Here's how the part is built. I have some questions about the finished solid (model axes, mm). Coordinates: 2 decimals unless noted, no trailing zeros. Write each loop counter-clockwise with the first axis right and the second up, starting at its lowest first coordinate (ties: lowest second). Pieces come first, ordered by that corner, then holes.
Item 1: We'd pull the mould along X, two halves only. Please class faces 1 (the face through (-10.84, 85.98, 48.81)), 2 (the face through (-34, 0, 33)), 3 (the face through (-45.471, 149.336, -13.573)): +X half, -X half, draft (parallel to the pull), parting line (faces both ways), or undercut.
Item 2: If I drill on line 1 (Z direction, x = 0, y = 46.5); line 2 (X direction, y = 38, z = 32), over which ranges is the centre line in solid material (lowest first)?
Item 3: If we section it at A-A (x = -41): Please give me the cut outline in (y, z).
Item 4: If we section it at B-B (y = 42): Please give me the cut outline in (x, z).
Item 5: I'm going to push flat-ended pins straight in: pin 1 Ø2 at (y, z) = (104.5, -22.5) entering from +X; pin 2 Ø1 at (y, z) = (104.5, -3.5) entering from +X; pin 3 Ø2 at (x, y) = (-13, 91.5) entering from +Z. Where does each tip first touch, or does it pass through?
Item 6: If we section it at C-C (x = 0): Please give me the cut outline in (y, z), then the cut area to 3 significant figures.
from build123d import *

# Parameters (mm, degrees)
EXTRUDE_1_OUTLINE_R      = 50
EXTRUDE_1_OUTLINE_R_2    = 47
EXTRUDE_1_DEPTH          = 200
CUT_EXTRUDE_1_DEPTH      = 213.132034356
CUT_EXTRUDE_1_DEPTH_BACK = 213.132034356
SKETCH_2_R               = 67.5


# Read off the part's stored shape, not the designer's step: Вытянуть-Тонкостенный1
with BuildPart() as part:
    # Вытянуть-Тонкостенный1 outline → Вытянуть-Тонкостенный1 (new body)
    with BuildSketch(Plane(origin=(0, 0, 0), x_dir=(1, 0, 0), z_dir=(0, 1, 0))):
        Circle(EXTRUDE_1_OUTLINE_R)
        Circle(EXTRUDE_1_OUTLINE_R_2, mode=Mode.SUBTRACT)
    extrude(amount=EXTRUDE_1_DEPTH)

    # Эскиз2 → Вырез-Вытянуть1 (cut, two sides: drawn at the far end of the back side and taken through both)
    with BuildSketch(Plane(origin=(0, 0, 0), x_dir=(1, 0, 0), z_dir=(0, -0.5735764363510444, -0.819152044288993)).offset(-CUT_EXTRUDE_1_DEPTH_BACK)):
        with Locations((0, -180)):
            Circle(SKETCH_2_R)
    extrude(amount=CUT_EXTRUDE_1_DEPTH + CUT_EXTRUDE_1_DEPTH_BACK, mode=Mode.SUBTRACT)


solid = part.part
Answer list:
1. face 1: parting line
1. face 2: draft
1. face 3: undercut
2. line 1: z = -50 to -47, 47 to 50
2. line 2: x = -38.42 to -34.42, 34.42 to 38.42
3. outline: (0, -28.62) - (134.24, -28.62) - (138.19, -22.98) - (0, -22.98) - close; (0, 22.98) - (170.37, 22.98) - (174.32, 28.62) - (0, 28.62) - close
4. outline: circle Ø100 at (0, 0); hole circle Ø94 at (0, 0)
5. pin 1: stops at x = 45.14
5. pin 2: stops at x = 49.91
5. pin 3: stops at z = 48.54
6. outline: (0, -50) - (102.33, -50) - (104.43, -47) - (0, -47) - close; (0, 47) - (170.25, 47) - (172.35, 50) - (0, 50) - close
6. area: 824 mm2
